The model under review builds one solid part; all positions refer to its coordinate system, in mm. Coordinates: 2 decimals unless noted, no trailing zeros. Loops run counter-clockwise (first coordinate to the right, second up) from the corner with the lowest first, then second, coordinate; pieces in that order, holes last. Notation, with made-up numbers: M -32,26.25 L 21,26.25 A27 ccw 21,54.25 Z; hole C -20,-27 d7. An arc over 180 degrees is marked long. Return JSON: item names as keys, results as strings.
```python
from build123d import *

# Parameters (mm, degrees)
SKETCH1_W           = 70
SKETCH1_H           = 55
BOSS_EXTRUDE1_DEPTH = 10
CHAMFER1_SIZE       = 1
M8_TAPPED_HOLE1_D   = 6.8
CHAMFER3_SIZE       = 1


with BuildPart() as part:
    # Sketch1 → Boss-Extrude1 (new body)
    with BuildSketch(Plane(origin=(0, 0, 0), x_dir=(1, 0, 0), z_dir=(0, 1, 0))):
        Rectangle(SKETCH1_W, SKETCH1_H)
    extrude(amount=-BOSS_EXTRUDE1_DEPTH)

    # Chamfer1
    chamfer1_edges = [part.edges().sort_by_distance(p)[0] for p in [
        (-35, -10, 0),
        (0, -10, 27.5),
        (35, -10, 0),
        (0, 0, 27.5),
        (-35, 0, 0),
        (0, 0, -27.5),
        (35, 0, 0),
        (0, -10, -27.5),
    ]]
    chamfer(chamfer1_edges, length=CHAMFER1_SIZE)

    # M8 Tapped Hole1 (through all)
    with Locations(Plane(origin=(0, 0, 0), x_dir=(1, 0, 0), z_dir=(0, 1, 0))):
        with Locations((0, 0)):
            Hole(M8_TAPPED_HOLE1_D / 2)

    # Chamfer3
    chamfer3_edges = [part.edges().sort_by_distance(p)[0] for p in [
        (35, -5, -27.5),
        (-35, -5, -27.5),
        (-35, -5, 27.5),
        (35, -5, 27.5),
    ]]
    chamfer(chamfer3_edges, length=CHAMFER3_SIZE)


solid = part.part
```
1. Add section A-A on z = 0. Give the boundary of the cut face in (x, y), plus the area to 3 significant figures.
Check values:
{"outline": "M -35,-9 L -34,-10 L -3.4,-10 L -3.4,0 L -34,0 L -35,-1 Z; M 3.4,-10 L 34,-10 L 35,-9 L 35,-1 L 34,0 L 3.4,0 Z", "area": "630 mm²"}
2. The part is to be moulded in two halves that separate along X. For faces 1 (the face through (35, -5, 0)), 2 (the face through (0, 0, -6)), 3 (the face through (0.74, -5.07, 3.32)), say which applies: released by +X, released by -X, zero draft, split by the parting line, or undercut.
Check values:
{"face 1": "released by +X", "face 2": "zero draft", "face 3": "undercut"}
3. To check wall thickness, follow line 1 (Z direction, x = 0, y = -5.5); line 2 (Z direction, x = 2, y = -6.5). State the ranges of each line that lie inside material, in increasing order.
Check values:
{"line 1": "-27.5 to -3.4, 3.4 to 27.5", "line 2": "-27.5 to -2.75, 2.75 to 27.5"}
4. Add section B-B on x = 0. Give the boundary of the cut face in (y, z).
Check values:
{"outline": "M -10,-26.5 L -9,-27.5 L -1,-27.5 L 0,-26.5 L 0,-3.4 L -10,-3.4 Z; M -10,3.4 L 0,3.4 L 0,26.5 L -1,27.5 L -9,27.5 L -10,26.5 Z"}
